Could you check a few things on this model? Use its own coordinates, in mm. Face numbers are marked on the shaded views. A direction names the side the tool comes from. Give positions to 0.01 mm unless a question says otherwise; leave off trailing zeros. Loops run counter-clockwise (first coordinate to the right, second up) from the corner with the lowest first, then second, coordinate; pieces in that order, holes last. Notation, with made-up numbers: (30, 22) - (85, 22) arc R21 ccw to (85, 49) - close; hole circle Ø10 at (15.5, 26). An arc over 180 degrees is marked (long way). Answer in a Markdown table with one row per item. Add a question column.
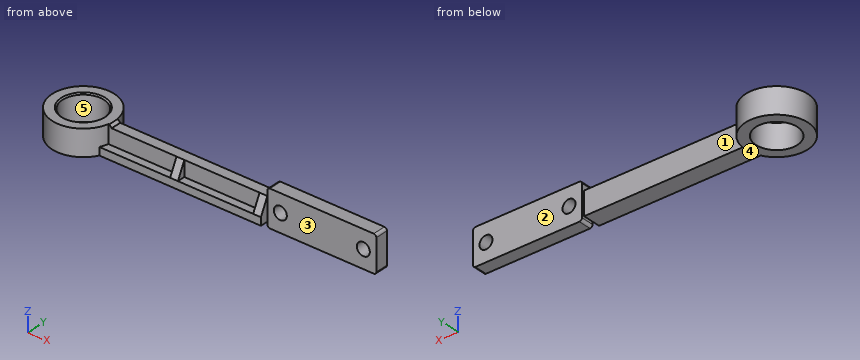
```python
from build123d import *

# Parameters (mm, degrees)
SKETCH_R        = 8
PAD_DEPTH       = 10
SKETCH001_R     = 2.5
POCKET_DEPTH    = 14.501
SKETCH002_W     = 42
SKETCH002_H     = 5
PAD001_DEPTH    = 2
SKETCH003_W     = 42
SKETCH003_H     = 5
PAD002_DEPTH    = 2
SKETCH004_W     = 62.22
SKETCH004_H     = 3
PAD003_DEPTH    = 3
PAD004_DEPTH    = 3
PAD005_DEPTH    = 3
FILLET_R        = 1
SKETCH007_W     = 60
SKETCH007_H     = 1
POCKET001_DEPTH = 14.501
CHAMFER_SIZE    = 0.95
CHAMFER001_SIZE = 0.5


with BuildPart() as part:
    # Sketch → Pad (new body)
    with BuildSketch(Plane.XY):
        with BuildLine():
            Line((0, 0), (-103.263305, 0))
            ThreePointArc((-103.094119, 4), (-126.98928, 3.007106), (-103.263305, 0))
            Line((-103.094119, 4), (-42, 4))
            Line((-42, 4), (-42, 5))
            Line((-42, 5), (0, 5))
            Line((0, 5), (0, 0))
        make_face()
        with Locations((-115, 2.5)):
            Circle(SKETCH_R, mode=Mode.SUBTRACT)
    extrude(amount=PAD_DEPTH)

    # Sketch001 (on Face1 of Pad) → Pocket (cut, through all)
    with BuildSketch(Plane.XZ):
        with Locations((-37, 5)):
            Circle(SKETCH001_R)
        with Locations((-5, 5)):
            Circle(SKETCH001_R)
    extrude(amount=-POCKET_DEPTH, mode=Mode.SUBTRACT)

    # Sketch002 (on Face4 of Pocket) → Pad001 (join)
    with BuildSketch(Plane.XY.offset(10)):
        with Locations((-21, 2.5)):
            Rectangle(SKETCH002_W, SKETCH002_H)
    extrude(amount=PAD001_DEPTH)

    # Sketch003 (on Face3 of Pad001) → Pad002 (join)
    with BuildSketch(Plane(origin=(0, 0, 0), x_dir=(1, 0, 0), z_dir=(0, 0, -1))):
        with Locations((-21, -2.5)):
            Rectangle(SKETCH003_W, SKETCH003_H)
    extrude(amount=PAD002_DEPTH)

    # Sketch004 → Pad003 (join)
    with BuildSketch(Plane.XZ):
        with Locations((-73.11, 1.5)):
            Rectangle(SKETCH004_W, SKETCH004_H)
    extrude(amount=PAD003_DEPTH)

    # Sketch005 → Pad004 (join)
    with BuildSketch(Plane.YZ.offset(-42)):
        Polygon((-3, 3), (0, 3), (0, 9), align=None)
    extrude(amount=-PAD004_DEPTH)

    # Sketch006 → Pad005 (join)
    with BuildSketch(Plane.YZ.offset(-74)):
        Polygon((-3, 3), (0, 3), (0, 9), align=None)
    extrude(amount=-PAD005_DEPTH)

    # Fillet
    fillet_edges = [part.edges().sort_by_distance(p)[0] for p in [
        (0, 2.5, -2),
        (0, 2.5, 12),
        (-42, 2.5, 12),
        (-42, 2.5, -2),
    ]]
    fillet(fillet_edges, radius=FILLET_R)

    # Sketch007 (on Face4 of Fillet) → Pocket001 (cut, through all)
    with BuildSketch(Plane.XZ):
        with Locations((-72, 9.5)):
            Rectangle(SKETCH007_W, SKETCH007_H)
    extrude(amount=-POCKET001_DEPTH, mode=Mode.SUBTRACT)

    # Chamfer
    chamfer_edges = [part.edges().sort_by_distance(p)[0] for p in [
        (-102, 2, 10),
    ]]
    chamfer(chamfer_edges, length=CHAMFER_SIZE)

    # Chamfer001
    chamfer001_edges = [part.edges().sort_by_distance(p)[0] for p in [
        (-123, 2.5, 10),
    ]]
    chamfer(chamfer001_edges, length=CHAMFER001_SIZE)


solid = part.part
```
(1) I want a section at C-C on x = -23. Please give me the cut outline in (y, z).
(2) I want a section at B-B on z = 6.25. Please give me the cut outline in (x, y) (3 decimals).
(3) For pin 1 Ø1.5 at (x, z) = (-16.5, 10.5) entering from +Y; pin 2 Ø0.9 at (y, z) = (-2, 4.5) entering from -X; pin 3 Ø2.5 at (y, z) = (-1, 5) entering from -X, each with a flat end and sliding along its axis, tell me the tip position at first contact or that it passes through.
(4) On a 3-axis mill with a long thin cutter (end or side, diameter ignored), from which of +Z, -Z, +X, -X, +Y, -Y can I reach the whole of each face in a straight line? I mean the marked faces 3, 4 and 5. Say none if no direction works.
(5) Please list where these lines run through material, in increasing order: line 1 (Z direction, x = -5, y = 4.05); line 2 (X direction, y = 4.25, z = 6); line 3 (X direction, y = 3.5, z = 3).
(6) I want a section at A-A on x = -5. Please give me the cut outline in (y, z).
(7) I want a section at D-D on x = -38. Please give me the cut outline in (y, z).
(8) We'd pull the mould along X, two halves only. Please class the marked faces 1 and 2: pulls with the +X half, pulls with the -X half, needs draft (parallel to the pull), parting line crosses it, or undercut.
Reported:
| question | item | result |
|---|---|---|
| 1 | outline | (0, -2) - (5, -2) - (5, 12) - (0, 12) - close |
| 2 | outline | (-103.263, 0) - (-77, 0) - (-77, -1.375) - (-74, -1.375) - (-74, 0) - (-45, 0) - (-45, -1.375) - (-42, -1.375) - (-42, 0) - (-39.165, 0) - (-39.165, 5) - (-42, 5) - (-42, 4) - (-103.094, 4) arc R12 ccw (long way) to start; (-34.835, 0) - (-7.165, 0) - (-7.165, 5) - (-34.835, 5) - close; (-2.835, 0) - (0, 0) - (0, 5) - (-2.835, 5) - close; hole circle Ø16 at (-115, 2.5) |
| 3 | pin 1 | y = 5 |
| 3 | pin 2 | x = -126.3 |
| 3 | pin 3 | x = -126.79 |
| 4 | face 3 | +Z, -Z, +X, -Y |
| 4 | face 4 | -Z, -X, +Y, -Y |
| 4 | face 5 | +Z, -Z |
| 5 | line 1 | -2 to 2.5, 7.5 to 12 |
| 5 | line 2 | -126.87 to -122.81, -107.19 to -103.13, -42 to -39.29, -34.71 to -7.29, -2.71 to 0 |
| 5 | line 3 | -126.96 to -122.94, -107.06 to -38.5, -35.5 to -6.5, -3.5 to 0 |
| 6 | outline | (0, -2) - (5, -2) - (5, 2.5) - (0, 2.5) - close; (0, 7.5) - (5, 7.5) - (5, 12) - (0, 12) - close |
| 7 | outline | (0, -2) - (5, -2) - (5, 2.71) - (0, 2.71) - close; (0, 7.29) - (5, 7.29) - (5, 12) - (0, 12) - close |
| 8 | face 1 | undercut |
| 8 | face 2 | needs draft |
